Model file for the job. Use its own axes, mm. A direction names the side the tool comes from. Round coordinates to 2 decimals unless told otherwise and drop trailing zeros. Loops run counter-clockwise (first coordinate to the right, second up) from the corner with the lowest first, then second, coordinate; pieces in that order, holes last. Notation, with made-up numbers: M 82.5,-40 L 123.5,-40 A30 ccw 123.5,-13 Z; hole C -37,47.25 d7. An arc over 180 degrees is marked long. Use a Markdown table: item, result. Add a question column.
Q1. Cut at A-A (z = 0). Give the cut face in (x, y), plus the area to 3 significant figures.
Q2. Cut at D-D (z = -16). Give the cut face in (x, y).
Q3. Mould opens along Y. For faces 1 (the face through (-49, 2, -4.965)), 2 (the face through (-1, 0, -8)), 3 (the face through (-75, 3, 11.066)) say: +Y half, -Y half, draft (parallel to the pull), parting line (faces both ways), or undercut.
Q4. Cut at C-C (x = -47). Give the cut face in (y, z), plus the area to 3 significant figures.
Q5. Cut at B-B (x = 66.5). Give the cut face in (y, z).
Q6. Tool access for faces 4 (the face through (-1, 3, -36.066)), 5 (the face through (65, 2, -14.013)): list every direction of +Z, -Z, +X, -X, +Y, -Y with a clear straight run to the whole face (end or side of a thin tool).
Q7. Pin check, flat tip, straight feed: pin 1 (1 mm diameter, centred on x = -75, y = 2.5, fed in from +Z). Stop position of the tip, or through.
Q8. Probe line 1 (Z direction, x = 61, y = 3.5); line 2 (Y direction, x = 75, z = 13); line 3 (X direction, y = 3.15, z = -16). List the from-to ranges inside material, lowest first. Write a range as from..to.
from build123d import *

# Parameters (mm, degrees)
SKETCH1_W           = 159.999999944
SKETCH1_H           = 42.132527592
BOSS_EXTRUDE1_DEPTH = 5
SKETCH4_R           = 1.6
CUT_EXTRUDE2_DEPTH  = 10
CUT_EXTRUDE4_DEPTH  = 6
SKETCH10_W          = 160
SKETCH10_H          = 10
BOSS_EXTRUDE4_DEPTH = 5
CUT_EXTRUDE5_DEPTH  = 6
SKETCH11_W          = 160
SKETCH11_H          = 5
BOSS_EXTRUDE5_DEPTH = 5


with BuildPart() as part:
    # Sketch1 → Boss-Extrude1 (new body)
    with BuildSketch(Plane(origin=(0, 0, 0), x_dir=(1, 0, 0), z_dir=(0, 1, 0))):
        Rectangle(SKETCH1_W, SKETCH1_H)
        with BuildLine():
            Line((-69.999999972, 18.546018972), (-59.999999972, 18.546018972))
            ThreePointArc((-59.999999972, 18.546018972), (-57.749999972, 16.296018972), (-59.999999972, 14.046018972))
            Line((-59.999999972, 14.046018972), (-69.999999972, 14.046018972))
            ThreePointArc((-69.999999972, 14.046018972), (-72.249999972, 16.296018972), (-69.999999972, 18.546018972))
        make_face(mode=Mode.SUBTRACT)
        with BuildLine():
            Line((-37.407962028, 18.546018972), (-27.407962028, 18.546018972))
            ThreePointArc((-27.407962028, 18.546018972), (-25.157962028, 16.296018972), (-27.407962028, 14.046018972))
            Line((-27.407962028, 14.046018972), (-37.407962028, 14.046018972))
            ThreePointArc((-37.407962028, 14.046018972), (-39.657962028, 16.296018972), (-37.407962028, 18.546018972))
        make_face(mode=Mode.SUBTRACT)
        with BuildLine():
            Line((-69.999999972, -18.546018972), (-59.999999972, -18.546018972))
            ThreePointArc((-59.999999972, -18.546018972), (-57.749999972, -16.296018972), (-59.999999972, -14.046018972))
            Line((-59.999999972, -14.046018972), (-69.999999972, -14.046018972))
            ThreePointArc((-69.999999972, -14.046018972), (-72.249999972, -16.296018972), (-69.999999972, -18.546018972))
        make_face(mode=Mode.SUBTRACT)
        with BuildLine():
            Line((-37.407962028, -18.546018972), (-27.407962028, -18.546018972))
            ThreePointArc((-27.407962028, -18.546018972), (-25.157962028, -16.296018972), (-27.407962028, -14.046018972))
            Line((-27.407962028, -14.046018972), (-37.407962028, -14.046018972))
            ThreePointArc((-37.407962028, -14.046018972), (-39.657962028, -16.296018972), (-37.407962028, -18.546018972))
        make_face(mode=Mode.SUBTRACT)
        with BuildLine():
            Line((-53.703981, 4.964699858), (-43.703981, 4.964699858))
            ThreePointArc((-43.703981, 4.964699858), (-38.739281142, 0), (-43.703981, -4.964699858))
            Line((-43.703981, -4.964699858), (-53.703981, -4.964699858))
            ThreePointArc((-53.703981, -4.964699858), (-58.668680858, 0), (-53.703981, 4.964699858))
        make_face(mode=Mode.SUBTRACT)
        with BuildLine():
            Line((37.440525033, 14.013455967), (27.440525033, 14.013455967))
            ThreePointArc((27.440525033, 14.013455967), (25.190525033, 16.263455967), (27.440525033, 18.513455967))
            Line((27.440525033, 18.513455967), (37.440525033, 18.513455967))
            ThreePointArc((37.440525033, 18.513455967), (39.690525033, 16.263455967), (37.440525033, 14.013455967))
        make_face(mode=Mode.SUBTRACT)
        with BuildLine():
            Line((69.967436967, 14.013455967), (59.967436967, 14.013455967))
            ThreePointArc((59.967436967, 14.013455967), (57.717436967, 16.263455967), (59.967436967, 18.513455967))
            Line((59.967436967, 18.513455967), (69.967436967, 18.513455967))
            ThreePointArc((69.967436967, 18.513455967), (72.217436967, 16.263455967), (69.967436967, 14.013455967))
        make_face(mode=Mode.SUBTRACT)
        with BuildLine():
            Line((53.703981, -5.050207727), (43.703981, -5.050207727))
            ThreePointArc((43.703981, -5.050207727), (38.653773273, 0), (43.703981, 5.050207727))
            Line((43.703981, 5.050207727), (53.703981, 5.050207727))
            ThreePointArc((53.703981, 5.050207727), (58.754188727, 0), (53.703981, -5.050207727))
        make_face(mode=Mode.SUBTRACT)
        with BuildLine():
            Line((37.440525033, -14.013455967), (27.440525033, -14.013455967))
            ThreePointArc((27.440525033, -14.013455967), (25.190525033, -16.263455967), (27.440525033, -18.513455967))
            Line((27.440525033, -18.513455967), (37.440525033, -18.513455967))
            ThreePointArc((37.440525033, -18.513455967), (39.690525033, -16.263455967), (37.440525033, -14.013455967))
        make_face(mode=Mode.SUBTRACT)
        with BuildLine():
            Line((69.967436967, -14.013455967), (59.967436967, -14.013455967))
            ThreePointArc((59.967436967, -14.013455967), (57.717436967, -16.263455967), (59.967436967, -18.513455967))
            Line((59.967436967, -18.513455967), (69.967436967, -18.513455967))
            ThreePointArc((69.967436967, -18.513455967), (72.217436967, -16.263455967), (69.967436967, -14.013455967))
        make_face(mode=Mode.SUBTRACT)
    extrude(amount=BOSS_EXTRUDE1_DEPTH)

    # Sketch4 → Cut-Extrude2 (cut)
    with BuildSketch(Plane.XY.offset(21.066263796)):
        with Locations((-74.999999972, 2.5)):
            Circle(SKETCH4_R)
        with Locations((74.999999972, 2.5)):
            Circle(SKETCH4_R)
        with Locations((0, 2.5)):
            Circle(SKETCH4_R)
    extrude(amount=-CUT_EXTRUDE2_DEPTH, mode=Mode.SUBTRACT)

    # Sketch9 → Cut-Extrude4 (cut, through all)
    with BuildSketch(Plane.XZ):
        with BuildLine():
            Line((2.070498026, -22.066263796), (2.070498026, -12.066263796))
            ThreePointArc((2.070498026, -12.066263796), (4.120498026, -10.016263796), (6.170498026, -12.066263796))
            Line((6.170498026, -12.066263796), (6.170498026, -22.066263796))
            ThreePointArc((6.170498026, -22.066263796), (4.120498026, -24.116263796), (2.070498026, -22.066263796))
        make_face()
    extrude(amount=-CUT_EXTRUDE4_DEPTH, mode=Mode.SUBTRACT)

    # Sketch10 → Boss-Extrude4 (add)
    with BuildSketch(Plane(origin=(0, 5, 0), x_dir=(1, 0, 0), z_dir=(0, 1, 0))):
        with Locations((2.8e-08, 26.066263796)):
            Rectangle(SKETCH10_W, SKETCH10_H)
    extrude(amount=-BOSS_EXTRUDE4_DEPTH)

    # Sketch9<2> → Cut-Extrude5 (cut, through all)
    with BuildSketch(Plane.XZ):
        with BuildLine():
            Line((2.070498026, -22.066263796), (2.070498026, -12.066263796))
            ThreePointArc((2.070498026, -12.066263796), (4.120498026, -10.016263796), (6.170498026, -12.066263796))
            Line((6.170498026, -12.066263796), (6.170498026, -22.066263796))
            ThreePointArc((6.170498026, -22.066263796), (4.120498026, -24.116263796), (2.070498026, -22.066263796))
        make_face()
    extrude(amount=-CUT_EXTRUDE5_DEPTH, mode=Mode.SUBTRACT)

    # Sketch11 → Boss-Extrude5 (add)
    with BuildSketch(Plane(origin=(0, 5, 0), x_dir=(1, 0, 0), z_dir=(0, 1, 0))):
        with Locations((2.8e-08, 33.566263796)):
            Rectangle(SKETCH11_W, SKETCH11_H)
    extrude(amount=-BOSS_EXTRUDE5_DEPTH)


solid = part.part
Checked values:
| question | item | result |
|---|---|---|
| 1 | outline | M -80,0 L -58.67,0 L -58.67,5 L -80,5 Z; M -38.74,0 L 38.65,0 L 38.65,5 L -38.74,5 Z; M 58.75,0 L 80,0 L 80,5 L 58.75,5 Z |
| 1 | area | 600 mm^2 |
| 2 | outline | M -80,0 L -72.23,0 L -72.23,5 L -80,5 Z; M -57.77,0 L -39.64,0 L -39.64,5 L -57.77,5 Z; M -25.18,0 L 2.07,0 L 2.07,5 L -25.18,5 Z; M 6.17,0 L 25.21,0 L 25.21,5 L 6.17,5 Z; M 39.68,0 L 57.73,0 L 57.73,5 L 39.68,5 Z; M 72.2,0 L 80,0 L 80,5 L 72.2,5 Z |
| 3 | face 1 | draft |
| 3 | face 2 | -Y half |
| 3 | face 3 | undercut |
| 4 | outline | M 0,-36.07 L 5,-36.07 L 5,-4.96 L 0,-4.96 Z; M 0,4.96 L 5,4.96 L 5,21.07 L 0,21.07 Z |
| 4 | area | 236 mm^2 |
| 5 | outline | M 0,-36.07 L 5,-36.07 L 5,-18.51 L 0,-18.51 Z; M 0,-14.01 L 5,-14.01 L 5,14.01 L 0,14.01 Z; M 0,18.51 L 5,18.51 L 5,21.07 L 0,21.07 Z |
| 6 | face 4 | -Z, +X, -X, +Y, -Y |
| 6 | face 5 | +Y, -Y |
| 7 | pin 1 | stops at z = 11.07 |
| 8 | line 1 | z = -36.07..-18.51, -14.01..14.01, 18.51..21.07 |
| 8 | line 2 | y = 0..0.9, 4.1..5 |
| 8 | line 3 | x = -80..-72.23, -57.77..-39.64, -25.18..2.07, 6.17..25.21, 39.68..57.73, 72.2..80 |
